Work out the finished part from the listing and answer in its coordinate system (mm). A direction names the side the tool comes from. Round coordinates to 2 decimals unless told otherwise and drop trailing zeros. Order: outer loops, then holes, each group sorted by start corner. A loop starts at its lowest first (then second) coordinate and runs counter-clockwise, first axis right, second up. Notation, with made-up numbers: (66, -33.5) - (97, -33.5) arc R27 cw to (97, -16.5) - close; hole circle Ø7 at (78, -2). An arc over 180 degrees is marked (long way). Use one line per item in the form item = value. Start each with the question number.
Q1. Which of the six approach directions +Z, -Z, +X, -X, +Y, -Y give full straight-line access (tool end or side, diameter ignored) to faces 1 (the flat face through (-4.677, 4.42, -6.091)), 2 (the flat face through (4, 4, 0)), 3 (the flat face through (-4, 4, 0))?
Q2. The part is cut by section A-A on z = 0. Determine the outline of the cut face in (x, y).
Q3. Given P1, Ø3, axis at x = -0.5, y = 9.5, coming from the +Z side; P2, Ø1.4, axis at x = 0, y = 2, coming from the -Z side; P3, Ø3, axis at x = -2, y = 18.5, coming from the -Z side, each flat-ended and moving along its own axis, determine where each tip first touches the part or whether it passes through.
Q4. The part is cut by section D-D on z = 5.5. Determine the outline of the cut face in (x, y).
Q5. The part is cut by section B-B on x = 0. Determine the outline of the cut face in (y, z).
Q6. Find the intervals of material crossed by line 1 (Z direction, x = 0, y = -4.5); line 2 (Z direction, x = 6, y = 9); line 3 (Z direction, x = 6.25, y = 14), in increasing order. Write a range as [from, to].
Q7. The part is cut by section C-C on x = -6. Determine the outline of the cut face in (y, z), plus the area to 3 significant figures.
Q8. For a pull along Z with two mould halves and no side action, classify faces 4 (the flat face through (6, 4, 10)), 5 (the flat face through (5, 4, -8)), 6 (the flat face through (10, 4, 7)) as +Z half, -Z half, draft (parallel to the pull), parting line (faces both ways), or undercut.
from build123d import *

# Parameters (mm, degrees)
SKETCH1_R           = 2
PROFILE_4X4_1_DEPTH = 60


with BuildPart() as part:
    # Sketch1 → Profile 4X4(1) (new body)
    with BuildSketch(Plane.XZ.offset(-34)):
        with BuildLine():
            Line((-3, 9.2), (-3, 8.8))
            ThreePointArc((-3, 8.8), (-3.234314575, 8.234314575), (-3.8, 8))
            Line((-3.8, 8), (-6.585786438, 8))
            Line((-6.585786438, 8), (-2.820101013, 4.234314575))
            ThreePointArc((-2.820101013, 4.234314575), (-2.560562334, 4.060896374), (-2.254415588, 4))
            Line((-2.254415588, 4), (2.254415588, 4))
            ThreePointArc((2.254415588, 4), (2.560562334, 4.060896374), (2.820101013, 4.234314575))
            Line((2.820101013, 4.234314575), (6.585786438, 8))
            Line((6.585786438, 8), (3.8, 8))
            ThreePointArc((3.8, 8), (3.234314575, 8.234314575), (3, 8.8))
            Line((3, 8.8), (3, 9.2))
            ThreePointArc((3, 9.2), (3.234314575, 9.765685425), (3.8, 10))
            Line((3.8, 10), (9.2, 10))
            ThreePointArc((9.2, 10), (9.765685425, 9.765685425), (10, 9.2))
            Line((10, 9.2), (10, 3.8))
            ThreePointArc((10, 3.8), (9.765685425, 3.234314575), (9.2, 3))
            Line((9.2, 3), (8.8, 3))
            ThreePointArc((8.8, 3), (8.234314575, 3.234314575), (8, 3.8))
            Line((8, 3.8), (8, 6.585786438))
            Line((8, 6.585786438), (4.234314575, 2.820101013))
            ThreePointArc((4.234314575, 2.820101013), (4.060896374, 2.560562334), (4, 2.254415588))
            Line((4, 2.254415588), (4, -2.254415588))
            ThreePointArc((4, -2.254415588), (4.060896374, -2.560562334), (4.234314575, -2.820101013))
            Line((4.234314575, -2.820101013), (8, -6.585786438))
            Line((8, -6.585786438), (8, -3.8))
            ThreePointArc((8, -3.8), (8.234314575, -3.234314575), (8.8, -3))
            Line((8.8, -3), (9.2, -3))
            ThreePointArc((9.2, -3), (9.765685425, -3.234314575), (10, -3.8))
            Line((10, -3.8), (10, -9.2))
            ThreePointArc((10, -9.2), (9.765685425, -9.765685425), (9.2, -10))
            Line((9.2, -10), (3.8, -10))
            ThreePointArc((3.8, -10), (3.234314575, -9.765685425), (3, -9.2))
            Line((3, -9.2), (3, -8.8))
            ThreePointArc((3, -8.8), (3.234314575, -8.234314575), (3.8, -8))
            Line((3.8, -8), (6.585786438, -8))
            Line((6.585786438, -8), (2.820101013, -4.234314575))
            ThreePointArc((2.820101013, -4.234314575), (2.560562334, -4.060896374), (2.254415588, -4))
            Line((2.254415588, -4), (-2.254415588, -4))
            ThreePointArc((-2.254415588, -4), (-2.560562334, -4.060896374), (-2.820101013, -4.234314575))
            Line((-2.820101013, -4.234314575), (-6.585786438, -8))
            Line((-6.585786438, -8), (-3.8, -8))
            ThreePointArc((-3.8, -8), (-3.234314575, -8.234314575), (-3, -8.8))
            Line((-3, -8.8), (-3, -9.2))
            ThreePointArc((-3, -9.2), (-3.234314575, -9.765685425), (-3.8, -10))
            Line((-3.8, -10), (-9.2, -10))
            ThreePointArc((-9.2, -10), (-9.765685425, -9.765685425), (-10, -9.2))
            Line((-10, -9.2), (-10, -3.8))
            ThreePointArc((-10, -3.8), (-9.765685425, -3.234314575), (-9.2, -3))
            Line((-9.2, -3), (-8.8, -3))
            ThreePointArc((-8.8, -3), (-8.234314575, -3.234314575), (-8, -3.8))
            Line((-8, -3.8), (-8, -6.585786438))
            Line((-8, -6.585786438), (-4.234314575, -2.820101013))
            ThreePointArc((-4.234314575, -2.820101013), (-4.060896374, -2.560562334), (-4, -2.254415588))
            Line((-4, -2.254415588), (-4, 2.254415588))
            ThreePointArc((-4, 2.254415588), (-4.060896374, 2.560562334), (-4.234314575, 2.820101013))
            Line((-4.234314575, 2.820101013), (-8, 6.585786438))
            Line((-8, 6.585786438), (-8, 3.8))
            ThreePointArc((-8, 3.8), (-8.234314575, 3.234314575), (-8.8, 3))
            Line((-8.8, 3), (-9.2, 3))
            ThreePointArc((-9.2, 3), (-9.765685425, 3.234314575), (-10, 3.8))
            Line((-10, 3.8), (-10, 9.2))
            ThreePointArc((-10, 9.2), (-9.765685425, 9.765685425), (-9.2, 10))
            Line((-9.2, 10), (-3.8, 10))
            ThreePointArc((-3.8, 10), (-3.234314575, 9.765685425), (-3, 9.2))
        make_face()
        Circle(SKETCH1_R, mode=Mode.SUBTRACT)
    extrude(amount=PROFILE_4X4_1_DEPTH)


solid = part.part
Found:
q1.face_1 = +Y, -Y
q1.face_2 = +X, +Y, -Y
q1.face_3 = -X, +Y, -Y
q2.outline = (-4, -26) - (-2, -26) - (-2, 34) - (-4, 34) - close; (2, -26) - (4, -26) - (4, 34) - (2, 34) - close
q3.P1 = 4
q3.P2 = -4
q3.P3 = -9.94
q4.outline = (-10, -26) - (-8, -26) - (-8, 34) - (-10, 34) - close; (-6.91, -26) - (-4.09, -26) - (-4.09, 34) - (-6.91, 34) - close; (4.09, -26) - (6.91, -26) - (6.91, 34) - (4.09, 34) - close; (8, -26) - (10, -26) - (10, 34) - (8, 34) - close
q5.outline = (-26, -4) - (34, -4) - (34, -2) - (-26, -2) - close; (-26, 2) - (34, 2) - (34, 4) - (-26, 4) - close
q6.line_1 = [-4, -2], [2, 4]
q6.line_2 = [-10, -8], [-7.41, -4.59], [4.59, 7.41], [8, 10]
q6.line_3 = [-10, -8], [-7.66, -4.84], [4.84, 7.66], [8, 10]
q7.outline = (-26, -10) - (34, -10) - (34, -8) - (-26, -8) - close; (-26, -7.41) - (34, -7.41) - (34, -4.59) - (-26, -4.59) - close; (-26, 4.59) - (34, 4.59) - (34, 7.41) - (-26, 7.41) - close; (-26, 8) - (34, 8) - (34, 10) - (-26, 10) - close
q7.area = 579 mm²
q8.face_4 = +Z half
q8.face_5 = undercut
q8.face_6 = draft
